Source: CAD feature listing. Evaluate the final solid. Frame: model axes, mm. A direction names the side the tool comes from. Round coordinates to 2 decimals unless told otherwise and drop trailing zeros. Order: outer loops, then holes, each group sorted by start corner. A loop starts at its lowest first (then second) coordinate and runs counter-clockwise, first axis right, second up. Notation, with made-up numbers: (67.25, -2.75) -> (80.25, -2.75) arc R7 cw to (80.25, 1.25) -> close; hole circle Ø2 at (26, 2). An arc over 180 degrees is marked (long way). Use a Markdown table: item, result. Add a question column.
```python
from build123d import *

# Parameters (mm, degrees)
SKETCH1_W               = 76.2
SKETCH1_H               = 35.56
BOSS_EXTRUDE1_DEPTH     = 63.5
SKETCH2_W               = 76.2
SKETCH2_H               = 10.16
CUT_EXTRUDE1_DEPTH      = 25.4
CUT_EXTRUDE2_DEPTH      = 10.16
CUT_EXTRUDE3_DEPTH      = 78.501223216
CUT_EXTRUDE3_DEPTH_BACK = 78.501223216


with BuildPart() as part:
    # Sketch1 → Boss-Extrude1 (new body)
    with BuildSketch(Plane(origin=(0, 0, 0), x_dir=(1, 0, 0), z_dir=(0, 1, 0))):
        Rectangle(SKETCH1_W, SKETCH1_H)
    extrude(amount=BOSS_EXTRUDE1_DEPTH)

    # Sketch2 → Cut-Extrude1 (cut)
    with BuildSketch(Plane(origin=(0, 63.5, 0), x_dir=(1, 0, 0), z_dir=(0, 1, 0))):
        Rectangle(SKETCH2_W, SKETCH2_H)
    extrude(amount=-CUT_EXTRUDE1_DEPTH, mode=Mode.SUBTRACT)

    # Sketch3 → Cut-Extrude2 (cut)
    with BuildSketch(Plane.XY.offset(-5.08)):
        Polygon((38.1, 7.62), (38.1, 38.1), (-38.1, 38.1), align=None)
    extrude(amount=CUT_EXTRUDE2_DEPTH, mode=Mode.SUBTRACT)

    # Sketch4 → Cut-Extrude3 (cut, two sides: drawn at the far end of the back side and taken through both)
    with BuildSketch(Plane(origin=(0, 0, 5.08), x_dir=(-1, 0, 0), z_dir=(0, 0, -1)).offset(-CUT_EXTRUDE3_DEPTH_BACK)):
        Polygon((38.1, 63.5), (-38.1, 33.02), (-38.1, 63.5), align=None)
    extrude(amount=CUT_EXTRUDE3_DEPTH + CUT_EXTRUDE3_DEPTH_BACK, mode=Mode.SUBTRACT)


solid = part.part
```
1) Section A-A on y = 52.5. Output: boundary loops of the cut face in (x, z).
2) Section C-C on y = 59. Output: boundary loops of the cut face in (x, z).
3) Section D-D on x = 13. Output: boundary loops of the cut face in (y, z).
4) Reachability of faces 1 (the flat face through (-1, 36, 5.08)), 2 (the flat face through (-0.53, 48.47, 11.52)) from +Z, -Z, +X, -X, +Y, -Y: full face, straight path, thin tool, end or side. Return the list, or none.
5) Section B-B on x = -33. Output: boundary loops of the cut face in (y, z), then the cut area to 3 significant figures.
6) First-contact query: pin 1 Ø2 at (x, z) = (-10, 2) entering from +Y; pin 2 Ø1.5 at (y, z) = (34.5, -4) entering from +X (3 decimals); pin 3 Ø2 at (y, z) = (34, -3.5) entering from +X. Flat tips, straight axial feed; report the tip coordinate or a pass-through.
7) Line query: probe 1 along Z at (x, y) = (-18, 41); probe 2 along Y at (x, z) = (35, 6.5); probe 3 along Y at (x, z) = (21.5, -5.5). Output: solid intervals per line, ascending. Write a range as from..to.
Conclusion:
| question | item | result |
|---|---|---|
| 1 | outline | (-38.1, -17.78) -> (-10.6, -17.78) -> (-10.6, -5.08) -> (-38.1, -5.08) -> close; (-38.1, 5.08) -> (-10.6, 5.08) -> (-10.6, 17.78) -> (-38.1, 17.78) -> close |
| 2 | outline | (-38.1, -17.78) -> (-26.85, -17.78) -> (-26.85, -5.08) -> (-38.1, -5.08) -> close; (-38.1, 5.08) -> (-26.85, 5.08) -> (-26.85, 17.78) -> (-38.1, 17.78) -> close |
| 3 | outline | (0, -17.78) -> (43.06, -17.78) -> (43.06, -5.08) -> (17.66, -5.08) -> (17.66, 5.08) -> (43.06, 5.08) -> (43.06, 17.78) -> (0, 17.78) -> close |
| 4 | face 1 | +X, +Y |
| 4 | face 2 | +Z, -Z, +X, +Y |
| 5 | outline | (0, -17.78) -> (61.46, -17.78) -> (61.46, -5.08) -> (36.06, -5.08) -> (36.06, 5.08) -> (61.46, 5.08) -> (61.46, 17.78) -> (0, 17.78) -> close |
| 5 | area | 1,930 mm^2 |
| 6 | pin 1 | stops at y = 27.26 |
| 6 | pin 2 | stops at x = -27.225 |
| 6 | pin 3 | stops at x = -25.35 |
| 7 | probe 1 | z = -17.78..-5.08, 5.08..17.78 |
| 7 | probe 2 | y = 0..34.26 |
| 7 | probe 3 | y = 0..39.66 |
